from build123d import *

# Parameters (mm, degrees)
F0_W = 13.434972614
F0_H = 20.8462406445


# Not quite as in the source:
# - ends of sketch curves that miss each other by under 0.0002 mm in the source are joined


with BuildPart() as f1:
    # F0 (on Front) → F1 (revolve)
    with BuildSketch(Plane.XZ):
        with BuildLine():
            ThreePointArc((31.0491894541, 4.37e-08), (37.0661020279, -6.0169125301), (43.0830146017, 4.37e-08))
            Line((43.0830146017, 4.37e-08), (31.0491894541, 4.37e-08))
        make_face()
        with Locations((54.5795354992, 10.4231199002)):
            Rectangle(F0_W, F0_H)
        with BuildLine():
            Line((31.0491894541, 4.37e-08), (43.0830146017, 4.37e-08))
            ThreePointArc((43.0830146017, 4.37e-08), (37.0661020279, 6.0169126175), (31.0491894541, 4.37e-08))
        make_face()
        with BuildLine():
            Line((47.8620491922, 20.8721738309), (0, 20.8721738309))
            Line((0, 20.8721738309), (0, 4.37e-08))
            Line((0, 4.37e-08), (4.3250534176, 4.37e-08))
            ThreePointArc((4.3250534176, 4.37e-08), (9.7163589671, 5.3913055932), (15.1076645166, 4.37e-08))
            Line((15.1076645166, 4.37e-08), (31.0491894541, 4.37e-08))
            ThreePointArc((31.0491894541, 4.37e-08), (37.0661020279, 6.0169126175), (43.0830146017, 4.37e-08))
            Line((43.0830146017, 4.37e-08), (47.8620491922, 4.37e-08))
            Line((47.8620491922, 4.37e-08), (47.8620491922, 20.8462402225))
            Line((47.8620491922, 20.8462402225), (47.8620491922, 20.8721738309))
        make_face()
        with BuildLine():
            ThreePointArc((15.1076645166, 4.37e-08), (9.7163589671, 5.3913055932), (4.3250534176, 4.37e-08))
            Line((4.3250534176, 4.37e-08), (15.1076645166, 4.37e-08))
        make_face()
        with BuildLine():
            Line((15.1076645166, 4.37e-08), (4.3250534176, 4.37e-08))
            ThreePointArc((4.3250534176, 4.37e-08), (9.7163589671, -5.3913055058), (15.1076645166, 4.37e-08))
        make_face()
    revolve(axis=Axis((0, 0, 10.4360869373), (0, 0, -1)))


solid = f1.part
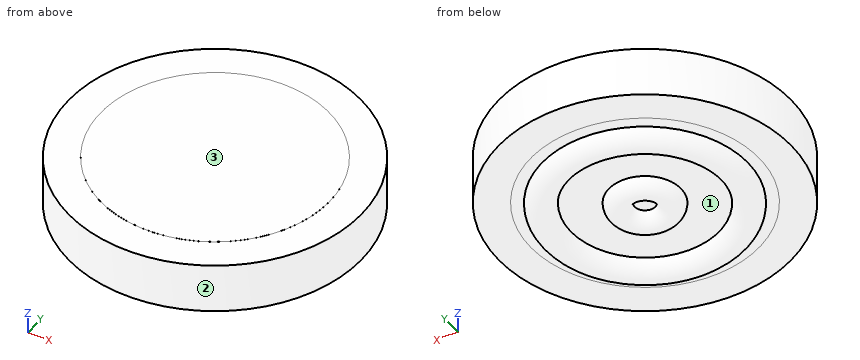
Build history of the part. All positions in model axes, mm. Face numbers are marked on the shaded views. Give positions to 0.01 mm unless a question says otherwise; leave off trailing zeros. Loops run counter-clockwise (first coordinate to the right, second up) from the corner with the lowest first, then second, coordinate; pieces in that order, holes last. Notation, with made-up numbers: (-22, 53.25) -> (14, 53.25) arc R28 ccw to (14, 72.25) -> close; hole circle Ø11 at (69.5, 43.5). An arc over 180 degrees is marked (long way). Answer in a Markdown table with one row per item.
Item 1: Slice it at C-C on z = 18.25. Write the cut outline in (x, y), plus the area to 3 significant figures.
Findings below:
| item | result |
|---|---|
| outline | circle Ø122.59 at (0, 0) |
| area | 11,800 mm² |
Item 2: Mould opens along Y. For the marked faces 1, 2 and 3 say: pulls with the +Y half, pulls with the -Y half, needs draft (parallel to the pull), parting line crosses it, or undercut.
Findings below:
| item | result |
|---|---|
| face 1 | undercut |
| face 2 | parting line crosses it |
| face 3 | needs draft |
Item 3: Flat gauge pins, fed straight in: P1, Ø4, axis at x = -44.5, y = -44.5, coming from the +Z side; P2, Ø1, axis at y = -44.5, z = 4.5, coming from the -X side; P3, Ø4, axis at y = 42.5, z = 14.5, coming from the +X side. Where does each tip first touch, or does it go through?
Findings below:
| item | result |
|---|---|
| P1 | stops at z = 20.85 |
| P2 | stops at x = -42.68 |
| P3 | stops at x = 46.01 |
Item 4: Probe line 1 along Y through (x, z) = (12, -3.75); line 2 along X through (y, z) = (-2.5, -0.5); line 3 along Z through (x, y) = (29.5, 48). List the from-to ranges inside material, lowest first. Write a range as [from, to].
Findings below:
| item | result |
|---|---|
| line 1 | y = [-40.01, -30.05], [-6.38, 6.38], [30.05, 40.01] |
| line 2 | x = [-42.99, -30.97], [-14.88, -3.56], [3.56, 14.88], [30.97, 42.99] |
| line 3 | z = [0, 20.85] |
